from build123d import *

# Parameters (mm, degrees)
SKETCH1_R           = 42.5
BOSS_EXTRUDE1_DEPTH = 10
SKETCH2_R           = 30
BOSS_EXTRUDE2_DEPTH = 30
SKETCH3_R           = 25.15
CUT_EXTRUDE1_DEPTH  = 73.197645391
CHAMFER1_SIZE       = 1
FILLET1_R           = 1
SKETCH4_R           = 2.25
CUT_EXTRUDE2_DEPTH  = 68.175144276
CIRPATTERN1_COUNT   = 6


with BuildPart() as part:
    # Sketch1 → Boss-Extrude1 (new body)
    with BuildSketch(Plane.XY):
        Circle(SKETCH1_R)
    extrude(amount=BOSS_EXTRUDE1_DEPTH)

    # Sketch2 → Boss-Extrude2 (add)
    with BuildSketch(Plane.XY.offset(10)):
        Circle(SKETCH2_R)
    extrude(amount=BOSS_EXTRUDE2_DEPTH)

    # Sketch3 → Cut-Extrude1 (cut, through all)
    with BuildSketch(Plane.XY.offset(40)):
        Circle(SKETCH3_R)
    extrude(amount=-CUT_EXTRUDE1_DEPTH, mode=Mode.SUBTRACT)

    # Chamfer1
    chamfer1_edges = [part.edges().sort_by_distance(p)[0] for p in [
        (-25.15, 0, 0),
        (-25.15, 0, 40),
    ]]
    chamfer(chamfer1_edges, length=CHAMFER1_SIZE)

    # Fillet1
    fillet1_edges = [part.edges().sort_by_distance(p)[0] for p in [
        (-42.5, 0, 10),
        (-30, 0, 10),
        (-30, 0, 40),
    ]]
    fillet(fillet1_edges, radius=FILLET1_R)

    # Sketch4 → Cut-Extrude2 (cut, through all)
    with BuildSketch(Plane.XY.offset(10)):
        with Locations((0, 35)):
            Circle(SKETCH4_R)
    cut_extrude2 = extrude(amount=-CUT_EXTRUDE2_DEPTH, mode=Mode.SUBTRACT)

    # CirPattern1: Cut-Extrude2 ×6 about axis
    cirpattern1_axis = Axis((0, 0, 0), (0, 0, 1))
    for i in range(1, CIRPATTERN1_COUNT):
        add(cut_extrude2.rotate(cirpattern1_axis, i * 360 / CIRPATTERN1_COUNT), mode=Mode.SUBTRACT)


solid = part.part
Input: part model. Units: mm. Frame: model coordinates. A direction names the side the tool comes from. Give positions to 0.01 mm unless a question says otherwise; leave off trailing zeros. Loops run counter-clockwise (first coordinate to the right, second up) from the corner with the lowest first, then second, coordinate; pieces in that order, holes last. Notation, with made-up numbers: (48.5, 2.25) - (68.5, 2.25) arc R25 cw to (68.5, 40.25) - close; hole circle Ø7 at (50.25, 88.5). An arc over 180 degrees is marked (long way). Use CSV: the item, a comma, the result in double quotes. Start each with the question number.
Item 1: Line query: line 1 (Y direction, x = 0, z = 2.75); line 2 (Y direction, x = 1, z = 26.5); line 3 (Z direction, x = 0.5, y = 31.5). Output: solid intervals per line, ascending.
Item 2: Contact query for flat-ended pins moving along their axis: P1, Ø1.5, axis at x = -15, z = 15, coming from the -Y side; P2, Ø7, axis at x = -30.31, y = 17.5, coming from the -Z side; P3, Ø3, axis at y = -6, z = 13.5, coming from the -X side; P4, Ø5, axis at x = 0, y = -35, coming from the +Z side. Output: stop coordinate, or through.
Item 3: Section B-B on y = 0. Return loops of the section in (x, z).
Item 4: Mould query, pull axis X, two halves, no side actions, for faces 1 (the flat face through (18.3, 19.5, 0)), 2 (the cylindrical face through (-29.97, 1.32, 24.8)), 3 (the cylindrical face through (-0.29, 37.23, 5.07)). Classes: pulls with the +X half, pulls with the -X half, needs draft (parallel to the pull), parting line crosses it, or undercut.
Item 5: Section A-A on x = 0. State how many separate pieces and enclosed holes the cut face has, then the cut area to 3 significant figures.
Item 6: Section C-C on z = 4. Return loops of the section in (x, y), then the cut area to 3 significant figures.
Item 7: Reachability of faces 4 (the flat face through (-6, -31, 10)), 5 (the cylindrical face through (32.096, 18.869, 5.07)) from +Z, -Z, +X, -X, +Y, -Y: full face, straight path, thin tool, end or side. Return the list, or none.
Item 8: Section D-D on z = 36. Return loops of the section in (x, y).
Ans:
1,line 1,"y = -42.5 to -37.25, -32.75 to -25.15, 25.15 to 32.75, 37.25 to 42.5"
1,line 2,"y = -29.98 to -25.13, 25.13 to 29.98"
1,line 3,"z = 0 to 10"
2,P1,"stops at y = -26.4"
2,P2,"stops at z = 0"
2,P3,"stops at x = -29.66"
2,P4,"stops at z = 10"
3,outline,"(-42.5, 0) - (-26.15, 0) - (-25.15, 1) - (-25.15, 39) - (-26.15, 40) - (-29, 40) arc R1 ccw to (-30, 39) - (-30, 11) arc R1 cw to (-31, 10) - (-41.5, 10) arc R1 ccw to (-42.5, 9) - close; (25.15, 1) - (26.15, 0) - (42.5, 0) - (42.5, 9) arc R1 ccw to (41.5, 10) - (31, 10) arc R1 cw to (30, 11) - (30, 39) arc R1 ccw to (29, 40) - (26.15, 40) - (25.15, 39) - close"
4,face 1,"needs draft"
4,face 2,"parting line crosses it"
4,face 3,"undercut"
5,separate pieces,"4"
5,enclosed holes,"0"
5,area,"546 mm2"
6,outline,"circle Ø85 at (0, 0); hole circle Ø4.5 at (-30.31, -17.5); hole circle Ø4.5 at (-30.31, 17.5); hole circle Ø50.3 at (0, 0); hole circle Ø4.5 at (0, -35); hole circle Ø4.5 at (0, 35); hole circle Ø4.5 at (30.31, -17.5); hole circle Ø4.5 at (30.31, 17.5)"
6,area,"3,590 mm2"
7,face 4,"+Z"
7,face 5,"+Z, -Z"
8,outline,"circle Ø60 at (0, 0); hole circle Ø50.3 at (0, 0)"
